Part model, mm, in its own coordinate system. A direction names the side the tool comes from. Coordinates: 2 decimals unless noted, no trailing zeros. Order: outer loops, then holes, each group sorted by start corner. A loop starts at its lowest first (then second) coordinate and runs counter-clockwise, first axis right, second up.
from build123d import *

# Parameters (mm, degrees)
F0_R     = 5.48
F1_DEPTH = 38.1
F2_T     = -0.8
F4_DEPTH = 19.05
F5_F1_R  = 0.100000054
F5_F2_R  = 0.100000054
F6_SIZE2 = 0.2886751346
F6_SIZE  = 0.5


with BuildPart() as f1:
    # F0 (on Top) → F1 (new body)
    with BuildSketch(Plane.XY):
        Circle(F0_R)
    extrude(amount=F1_DEPTH)

    # F2
    f2_openings = [f1.faces().sort_by_distance(p)[0] for p in [
        (0, 0, 38.1),
    ]]
    offset(amount=F2_T, openings=f2_openings)

    # F3 (on face) → F4 (cut)
    with BuildSketch(Plane.XY.offset(38.1)):
        with BuildLine():
            Line((0.508, 4.6523473645), (0.508, 5.4564032109))
            ThreePointArc((0.508, 5.4564032109), (0, 5.48), (-0.508, 5.4564032109))
            Line((-0.508, 5.4564032109), (-0.508, 4.6523473645))
            ThreePointArc((-0.508, 4.6523473645), (0, 4.68), (0.508, 4.6523473645))
        make_face()
        with BuildLine():
            Line((0.508, -5.4564032109), (0.508, -4.6523473645))
            ThreePointArc((0.508, -4.6523473645), (0, -4.68), (-0.508, -4.6523473645))
            Line((-0.508, -4.6523473645), (-0.508, -5.4564032109))
            ThreePointArc((-0.508, -5.4564032109), (0, -5.48), (0.508, -5.4564032109))
        make_face()
    extrude(amount=-F4_DEPTH, mode=Mode.SUBTRACT)

    # F5: fillet of radius 0.100000054 on 20 edges, made by hand

    # F5_f1
    f5_f1_edges = [f1.edges().sort_by_distance(p)[0] for p in [
        (0.508, -5.0543752877, 19.05),
        (-0.508, -5.0543752877, 19.05),
        (-0.508, 5.0543752877, 19.05),
        (0.508, 5.0543752877, 19.05),
    ]]
    fillet(f5_f1_edges, radius=F5_F1_R)

    # F5_f2
    f5_f2_edges = [f1.edges().sort_by_distance(p)[0] for p in [
        (-0.508, 5.0543752877, 38.1),
        (-4.68, 0, 38.1),
        (-0.508, -5.0543752877, 38.1),
        (-5.48, 0, 38.1),
        (4.0505703302, -3.6909727715, 38.1),
        (0.508, -5.0543752877, 38.1),
        (3.4842387978, -3.1244967595, 38.1),
        (3.4842387978, 3.1244967595, 38.1),
        (0.508, 5.0543752877, 38.1),
        (4.0505703302, 3.6909727715, 38.1),
        (0.508, -5.4564032109, 28.625000027),
        (0.508, -4.6523473645, 28.625000027),
        (-0.508, -4.6523473645, 28.625000027),
        (-0.508, -5.4564032109, 28.625000027),
        (0, 4.68, 19.05),
        (0, 5.48, 19.05),
        (0.4787933813, 5.4590435891, 19.0793721529),
        (-0.4787933846, 5.4590435887, 19.0793721564),
        (-0.4787918965, 4.6554439453, 19.0793706648),
        (0.4787918943, 4.6554439457, 19.0793706623),
        (-0.4787933813, -5.4590435891, 19.0793721529),
        (-0.4787918943, -4.6554439457, 19.0793706623),
        (0.4787918943, -4.6554439457, 19.0793706623),
        (0.4787933813, -5.4590435891, 19.0793721529),
    ]]
    fillet(f5_f2_edges, radius=F5_F2_R)

    # F6
    f6_edges = [f1.edges().sort_by_distance(p)[0] for p in [
        (-5.48, 0, 0),
    ]]
    f6_side = f1.faces().sort_by_distance((-5.48, 0, 19))[0]
    chamfer(f6_edges, length=F6_SIZE, length2=F6_SIZE2, reference=f6_side)


solid = f1.part
Q1. Cut at D-D on z = 17. Write the cut outline in (x, y).
Results list:
outline: circle Ø10.96 at (0, 0); hole circle Ø9.36 at (0, 0)
Q2. Cut at B-B on x = 0. Write the cut outline in (y, z), and give its area (3 significant figures).
Results list:
outline: (-5.48, 0.5) - (-5.19, 0) - (5.19, 0) - (5.48, 0.5) - (5.48, 18.95) arc R0.1 ccw to (5.38, 19.05) - (4.78, 19.05) arc R0.1 ccw to (4.68, 18.95) - (4.68, 0.8) - (-4.68, 0.8) - (-4.68, 18.95) arc R0.1 ccw to (-4.78, 19.05) - (-5.38, 19.05) arc R0.1 ccw to (-5.48, 18.95) - close
area: 37.8 mm2
Q3. Pin check, flat tips, straight feed: pin 1 Ø1.5 at (y, z) = (-4, 31.5) entering from +X; pin 2 Ø0.5 at (y, z) = (-5, 28) entering from +X; pin 3 Ø1 at (x, z) = (2, 27.5) entering from +Y. Stop position of each tip, or through.
Results list:
pin 1: stops at x = 4.41
pin 2: stops at x = 2.73
pin 3: stops at y = 5.27
Q4. Mould opens along Y. For faces 3 (the face through (-3.71, -2.85, 19.14)), 4 (the face through (0, 0, 0)), 5 (the face through (5.227, 1.646, 18.987)) say: pulls with the +Y half, pulls with the -Y half, needs draft (parallel to the pull), parting line crosses it, or undercut.
Results list:
face 3: undercut
face 4: needs draft
face 5: parting line crosses it
Q5. Cut at C-C on y = 0. Write the cut outline in (x, z), and give its area (3 significant figures).
Results list:
outline: (-5.48, 0.5) - (-5.19, 0) - (5.19, 0) - (5.48, 0.5) - (5.48, 38) arc R0.1 ccw to (5.38, 38.1) - (4.78, 38.1) arc R0.1 ccw to (4.68, 38) - (4.68, 0.8) - (-4.68, 0.8) - (-4.68, 38) arc R0.1 ccw to (-4.78, 38.1) - (-5.38, 38.1) arc R0.1 ccw to (-5.48, 38) - close
area: 68.3 mm2
Q6. Which spindle directions (+Z, -Z, +X, -X, +Y, -Y) get a long thin tool onto all of the face, cutting with end or side? Do faces 1 (the face through (5, 1, 38.1)), 2 (the face through (0, 0, 0.8)). Say none if no direction does.
Results list:
face 1: +Z, +X, -X, +Y, -Y
face 2: +Z
Q7. Wall check: line 1 along Y through (x, z) = (0, 18.5); line 2 along X through (y, z) = (-1.25, 32); line 3 along X through (y, z) = (3.75, 16). Give the ranges that are in metal, low to high.
Results list:
line 1: y = -5.48 to -4.68, 4.68 to 5.48
line 2: x = -5.34 to -4.51, 4.51 to 5.34
line 3: x = -4 to -2.8, 2.8 to 4
